Build history of the part. All positions in model axes, mm. Round coordinates to 2 decimals unless told otherwise and drop trailing zeros. Loops run counter-clockwise (first coordinate to the right, second up) from the corner with the lowest first, then second, coordinate; pieces in that order, holes last. Notation, with made-up numbers: (-25.5, 64) - (-17.5, 64) arc R20 ccw to (-17.5, 75) - close; hole circle Ø10 at (4.5, 40.5). An arc over 180 degrees is marked (long way). Use one line per item in the form item = value. Start each with the question number.
Q1. Pin check, flat tips, straight feed: pin 1 (6.5 mm diameter, centred on x = 58.5, y = -20, fed in from +Z); pin 2 (9 mm diameter, centred on x = 58.5, y = 20, fed in from +Z); pin 3 (10 mm diameter, centred on x = 37, y = 6, fed in from -Z). Stop position of each tip, or through.
Q2. Mould opens along Y. For faces 1 (the face through (55.773, -19.642, 0.616)), 2 (the face through (58.6, -17.1, 1.4)), 3 (the face through (-1, 32.5, 2)), 4 (the face through (1, -32.5, 2)) say: released by +Y, released by -Y, zero draft, split by the parting line, or undercut.
Q3. Saw through at C-C (x = 58.5). Give the cut face in (y, z), then the cut area to 3 significant figures.
Q4. Saw through at B-B (z = 2.45). Give the cut face in (x, y).
Q5. Saw through at A-A (y = 20). Give the cut face in (x, z).
Q6. Drill centre lines: line 1 (X direction, y = 20, z = 0.3); line 2 (Y direction, x = 58.5, z = 0.9); line 3 (X direction, y = 22.5, z = 1.5). Where is each one in solid material? Low to high.
Autodesk Inventor part; units mm, degrees
ref_plane "YZ Plane" through (0, 0, 0) normal (1, 0, 0) x (0, 1, 0)
ref_plane "XZ Plane" through (0, 0, 0) normal (0, 1, 0) x (-1, 0, 0)
ref_plane "XY Plane" through (0, 0, 0) normal (0, 0, 1) x (1, 0, 0)
sketch "Sketch5" plane through (0, 0, 0) normal (0, 0, 1) x (1, 0, 0)
  line L0 (-65, 32.5) -> (65, 32.5)
  line L1 (65, 32.5) -> (65, -32.5)
  line L2 (65, -32.5) -> (-65, -32.5)
  line L3 (-65, -32.5) -> (-65, 32.5)
  point P0 (0, 0)
  point P1 (0, 32.5)
  point P2 (65, 0)
  dimension "d8" = 130
  dimension "d9" = 65
extrude "Extrusion5" add sketch "Sketch5" along normal blind 4
sketch "Sketch6" plane through (0, 0, 4) normal (0, 0, 1) x (1, 0, 0)
  circle A0 centre (-58.5, 20) radius 3
  circle A1 centre (-58.5, -20) radius 3
  circle A2 centre (58.5, 20) radius 3
  circle A3 centre (58.5, -20) radius 3
  point P0 (0, 0)
  point P1 (0, 0)
  dimension "d19" = 117
  dimension "d20" = 58.5
  dimension "d21" = 40
  dimension "d22" = 20
  dimension "d23" = 6
hole "Hole1" at (-58.5, 20, 4) at (58.5, 20, 4) at (58.5, -20, 4) at (-58.5, -20, 4) direction (0, 0, -1) diameter 5.5 end through all countersink diameter 11 countersink angle 90
chamfer "Chamfer1" distance 2 angle 45 4 edges at (65, 32.5, 2) (65, -32.5, 2) (-65, -32.5, 2) (-65, 32.5, 2)
properties part number "BC-10024" material "Alumínio 7075"
Report:
q1.pin_1 = 1.75
q1.pin_2 = 3
q1.pin_3 = 0
q2.face_1 = undercut
q2.face_2 = undercut
q2.face_3 = released by +Y
q2.face_4 = released by -Y
q3.outline = (-32.5, 0) - (-22.75, 0) - (-22.75, 1.25) - (-25.5, 4) - (-32.5, 4) - close; (-17.25, 0) - (17.25, 0) - (17.25, 1.25) - (14.5, 4) - (-14.5, 4) - (-17.25, 1.25) - close; (22.75, 0) - (32.5, 0) - (32.5, 4) - (25.5, 4) - (22.75, 1.25) - close
q3.area = 201 mm²
q4.outline = (-65, -30.5) - (-63, -32.5) - (63, -32.5) - (65, -30.5) - (65, 30.5) - (63, 32.5) - (-63, 32.5) - (-65, 30.5) - close; hole circle Ø7.9 at (-58.5, -20); hole circle Ø7.9 at (-58.5, 20); hole circle Ø7.9 at (58.5, -20); hole circle Ø7.9 at (58.5, 20)
q5.outline = (-65, 0) - (-61.25, 0) - (-61.25, 1.25) - (-64, 4) - (-65, 4) - close; (-55.75, 0) - (55.75, 0) - (55.75, 1.25) - (53, 4) - (-53, 4) - (-55.75, 1.25) - close; (61.25, 0) - (65, 0) - (65, 4) - (64, 4) - (61.25, 1.25) - close
q6.line_1 = -65 to -61.25, -55.75 to 55.75, 61.25 to 65
q6.line_2 = -32.5 to -22.75, -17.25 to 17.25, 22.75 to 32.5
q6.line_3 = -65 to -60.16, -56.84 to 56.84, 60.16 to 65
